Could you check a few things on this model? Use its own coordinates, in mm. Round coordinates to 2 decimals unless told otherwise and drop trailing zeros. Loops run counter-clockwise (first coordinate to the right, second up) from the corner with the lowest first, then second, coordinate; pieces in that order, holes last. Notation, with made-up numbers: (71.25, -10.5) -> (95.25, -10.5) arc R35 cw to (95.25, 25.5) -> close; hole circle Ø8 at (64.5, -16). An arc over 180 degrees is marked (long way). Write each question's results on one line, items separated by ' | '.
from build123d import *

# Parameters (mm, degrees)
SKETCH3_W                      = 203.2
SKETCH3_H                      = 6.35
BOSS_EXTRUDE1_DEPTH            = 76.2
BOSS_EXTRUDE1_DEPTH_BACK       = 76.2
F_3_8_16_TAPPED_HOLE1_D        = 7.9375
F_3_8_16_TAPPED_HOLE1_DEPTH    = 6.35
F_1_4_0_2500_DOWEL_HOLE1_D     = 6.35
F_1_4_0_2500_DOWEL_HOLE1_DEPTH = 6.35
F_3_8_16_TAPPED_HOLE2_D        = 7.9375
F_3_8_16_TAPPED_HOLE2_DEPTH    = 6.35
SKETCH10_W                     = 203.2
SKETCH10_H                     = 12.7
CUT_EXTRUDE1_DEPTH             = 7.35
FILLET1_R                      = 6.35


with BuildPart() as part:
    # Sketch3 → Boss-Extrude1 (new body, two sides)
    with BuildSketch(Plane.XY) as boss_extrude1_sk:
        Rectangle(SKETCH3_W, SKETCH3_H)
    extrude(amount=BOSS_EXTRUDE1_DEPTH)
    extrude(boss_extrude1_sk.sketch, amount=-BOSS_EXTRUDE1_DEPTH_BACK)

    # 3/8-16 Tapped Hole1
    with Locations(Plane(origin=(0, 3.175, 0), x_dir=(1, 0, 0), z_dir=(0, 1, 0))):
        with Locations((-76.2, -63.5), (-25.4, -63.5), (25.4, -63.5), (76.2, -63.5), (-25.4, -25.4), (25.4, -25.4), (76.2, -25.4), (-25.4, 12.7), (25.4, 12.7), (76.2, 12.7), (-25.4, 50.8), (25.4, 50.8), (76.2, 50.8), (-76.2, -25.4), (-76.2, 12.7), (-76.2, 50.8)):
            Hole(F_3_8_16_TAPPED_HOLE1_D / 2, depth=F_3_8_16_TAPPED_HOLE1_DEPTH)

    # 1/4 (0.2500) Dowel Hole1
    with Locations(Plane(origin=(0, 3.175, 0), x_dir=(1, 0, 0), z_dir=(0, 1, 0))):
        with Locations((-50.8, -63.5), (0, -63.5), (50.8, -63.5), (0, -25.4), (50.8, -25.4), (0, 12.7), (50.8, 12.7), (0, 50.8), (50.8, 50.8), (-50.8, -25.4), (-50.8, 12.7), (-50.8, 50.8)):
            Hole(F_1_4_0_2500_DOWEL_HOLE1_D / 2, depth=F_1_4_0_2500_DOWEL_HOLE1_DEPTH)

    # 3/8-16 Tapped Hole2
    with Locations(Plane(origin=(0, 3.175, 0), x_dir=(1, 0, 0), z_dir=(0, 1, 0))):
        with Locations((-88.9, 31.75), (-88.9, -44.45), (88.9, -44.45), (88.9, 31.75)):
            Hole(F_3_8_16_TAPPED_HOLE2_D / 2, depth=F_3_8_16_TAPPED_HOLE2_DEPTH)

    # Sketch10 → Cut-Extrude1 (cut, through all)
    with BuildSketch(Plane(origin=(0, 3.175, 0), x_dir=(1, 0, 0), z_dir=(0, 1, 0))):
        with Locations((0, 69.85)):
            Rectangle(SKETCH10_W, SKETCH10_H)
    extrude(amount=-CUT_EXTRUDE1_DEPTH, mode=Mode.SUBTRACT)

    # Fillet1
    fillet1_edges = [part.edges().sort_by_distance(p)[0] for p in [
        (101.6, 0, 76.2),
        (-101.6, 0, -63.5),
        (101.6, 0, -63.5),
        (-101.6, 0, 76.2),
    ]]
    fillet(fillet1_edges, radius=FILLET1_R)


solid = part.part
1) I'm going to push flat-ended pins straight in: pin 1 (6.5 mm diameter, centred on x = 76.2, z = -12.7, fed in from +Y); pin 2 (10.5 mm diameter, centred on x = 25.4, z = 63.5, fed in from +Y) (3 decimals). Where does each tip first touch, or does it pass through?
Model answer:
pin 1: passes through | pin 2: stops at y = 3.175
2) I need wall thicknesses on line 1 (Z direction, x = -25.4, y = -1.5); line 2 (Z direction, x = -26, y = -1.5); line 3 (X direction, y = -1.75, z = 44.45). Which ranges of each line are inside material? Lowest first, please.
Model answer:
line 1: z = -63.5 to -54.77, -46.83 to -16.67, -8.73 to 21.43, 29.37 to 59.53, 67.47 to 76.2 | line 2: z = -63.5 to -54.72, -46.88 to -16.62, -8.78 to 21.48, 29.32 to 59.58, 67.42 to 76.2 | line 3: x = -101.6 to -92.87, -84.93 to 84.93, 92.87 to 101.6
3) I want a section at A-A, the plane x = -25.4. Write out the boundary of the cut face in (y, z) (3 decimals), plus the area to 3 significant figures.
Model answer:
outline: (-3.175, -63.5) -> (3.175, -63.5) -> (3.175, -54.769) -> (-3.175, -54.769) -> close; (-3.175, -46.831) -> (3.175, -46.831) -> (3.175, -16.669) -> (-3.175, -16.669) -> close; (-3.175, -8.731) -> (3.175, -8.731) -> (3.175, 21.431) -> (-3.175, 21.431) -> close; (-3.175, 29.369) -> (3.175, 29.369) -> (3.175, 59.531) -> (-3.175, 59.531) -> close; (-3.175, 67.469) -> (3.175, 67.469) -> (3.175, 76.2) -> (-3.175, 76.2) -> close | area: 685 mm2
4) I want a section at B-B, the plane z = -12.7. Give the number of separate pieces and of enclosed holes in the cut face, plus the area to 3 significant figures.
Model answer:
separate pieces: 8 | enclosed holes: 0 | area: 968 mm2
5) I want a section at C-C, the plane x = 88.9. Write out the boundary of the cut face in (y, z) (3 decimals).
Model answer:
outline: (-3.175, -63.5) -> (3.175, -63.5) -> (3.175, -35.719) -> (-3.175, -35.719) -> close; (-3.175, -27.781) -> (3.175, -27.781) -> (3.175, 40.481) -> (-3.175, 40.481) -> close; (-3.175, 48.419) -> (3.175, 48.419) -> (3.175, 76.2) -> (-3.175, 76.2) -> close
6) If we mould it in two halves opening along X, with no side actions, what happens to faces 1 (the flat face through (-101.6, 0, 7)), 2 (the cylindrical face through (-1.707, -0.044, 60.823)), 3 (the flat face through (101.6, 0, 7))? For each: released by +X, released by -X, zero draft, split by the parting line, or undercut.
Model answer:
face 1: released by -X | face 2: undercut | face 3: released by +X
7) I want a section at D-D, the plane z = -31.75. Write out the boundary of the cut face in (x, y) (3 decimals).
Model answer:
outline: (-101.6, -3.175) -> (-92.869, -3.175) -> (-92.869, 3.175) -> (-101.6, 3.175) -> close; (-84.931, -3.175) -> (84.931, -3.175) -> (84.931, 3.175) -> (-84.931, 3.175) -> close; (92.869, -3.175) -> (101.6, -3.175) -> (101.6, 3.175) -> (92.869, 3.175) -> close
